Geometry check sheet. Reference: drawing and pictorial views, mm from the part's lowest x, y, z. Coordinates: 2 decimals unless noted, no trailing zeros. Loops run counter-clockwise (first coordinate to the right, second up) from the corner with the lowest first, then second, coordinate; pieces in that order, holes last. Notation, with made-up numbers: (-21, -4) - (7, -4) arc R9 cw to (7, 4) - close; hole circle Ø7 at (22.25, 55). An arc over 180 degrees is marked (long way). One line per item, written item: value.
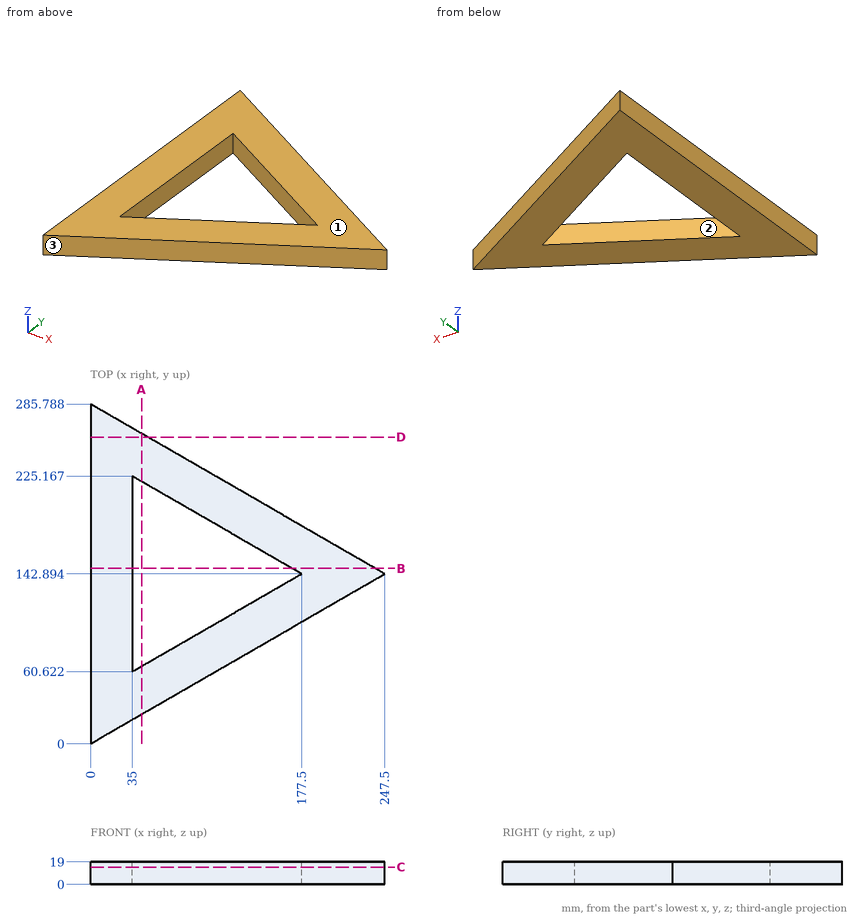
(1) Cross-section at C-C on z = 14.5. Record the cut outline in (x, y), and give its area (3 significant figures).
Reply:
outline: (0, 0) - (247.5, 142.89) - (0, 285.79) - close; hole (35, 60.62) - (177.5, 142.89) - (35, 225.17) - close
area: 23,600 mm2
(2) Cross-section at A-A on x = 43. Record the cut outline in (y, z), and give its area (3 significant figures).
Reply:
outline: (24.83, 0) - (65.24, 0) - (65.24, 19) - (24.83, 19) - close; (220.55, 0) - (260.96, 0) - (260.96, 19) - (220.55, 19) - close
area: 1,540 mm2
(3) Material ranges on probe 1 along X at (y, z) = (181, 12.75); probe 2 along X at (y, z) = (104, 10) (1 decimal); probe 3 along Y at (x, z) = (162, 11) (1 decimal), recorded low to high. Write a range as from..to.
Reply:
probe 1: 0..35, 111.5..181.5
probe 2: 0..35, 110.1..180.1
probe 3: 93.5..133.9, 151.8..192.3
(4) Cross-section at B-B on y = 147.5. Record the cut outline in (x, z).
Reply:
outline: (0, 0) - (35, 0) - (35, 19) - (0, 19) - close; (169.52, 0) - (239.52, 0) - (239.52, 19) - (169.52, 19) - close
(5) Cross-section at D-D on y = 258. Record the cut outline in (x, z).
Reply:
outline: (0, 0) - (48.13, 0) - (48.13, 19) - (0, 19) - close
(6) Go/stop test with flat-tipped pins: pin 1 Ø3 at (x, z) = (138.5, 2.5) entering from +Y; pin 2 Ø9.5 at (y, z) = (125.5, 10) entering from +X; pin 3 Ø2 at (x, z) = (213.5, 12) entering from +Y. Record where each tip stops, or that it passes through.
Reply:
pin 1: y = 206.69
pin 2: x = 225.6
pin 3: y = 163.1
(7) Release check for a two-part mould opening along Y. For the marked faces 1, 2 and 3 record: pulls with the +Y half, pulls with the -Y half, needs draft (parallel to the pull), parting line crosses it, or undercut.
Reply:
face 1: needs draft
face 2: undercut
face 3: pulls with the -Y half
